The listing builds one solid part. Answer for the finished solid, in the listing's coordinates (mm). A direction names the side the tool comes from. Coordinates: 2 decimals unless noted, no trailing zeros. Order: outer loops, then holes, each group sorted by start corner. A loop starts at its lowest first (then second) coordinate and runs counter-clockwise, first axis right, second up. Notation, with made-up numbers: (-19, -5.75) -> (33, -5.75) arc R21 ccw to (33, 1.25) -> close; hole circle Ø8 at (-32.75, -18.5). An arc over 180 degrees is marked (long way). Return JSON: item names as keys, results as strings.
from build123d import *

# Parameters (mm, degrees)
F0_R     = 6
F1_DEPTH = 120
F2_R     = 3.5
F3_DEPTH = 20
F5_SIZE  = 1
F6_SIZE  = 0.5
F7_W     = 7
F7_H     = 2.68
F8_DEPTH = 12.5


with BuildPart() as f1:
    # F0 (on Front) → F1 (new body)
    with BuildSketch(Plane.XZ):
        Circle(F0_R)
    extrude(amount=F1_DEPTH)

    # F2 (on face) → F3 (cut)
    with BuildSketch(Plane.XZ.offset(120)):
        Circle(F2_R)
    extrude(amount=-F3_DEPTH, mode=Mode.SUBTRACT)

    # F5
    f5_edges = [f1.edges().sort_by_distance(p)[0] for p in [
        (-6, 0, 0),
    ]]
    chamfer(f5_edges, length=F5_SIZE)

    # F6
    f6_edges = [f1.edges().sort_by_distance(p)[0] for p in [
        (-6, -120, 0),
    ]]
    chamfer(f6_edges, length=F6_SIZE)

    # F7 (on Right) → F8 (cut, symmetric)
    with BuildSketch(Plane.YZ):
        with Locations((-96.5, 1.34)):
            Rectangle(F7_W, F7_H)
        with Locations((-96.5, -1.34)):
            Rectangle(F7_W, F7_H)
    extrude(amount=F8_DEPTH, both=True, mode=Mode.SUBTRACT)


solid = f1.part
1. For faces 4 (the face through (0, 0, 0)), 5 (the face through (0, -97, 2.68)), determine the directions among +Z, -Z, +X, -X, +Y, -Y from which every point of the face is accessible in a straight line to the end or side of a thin tool.
Answer block:
{"face 4": "+Z, -Z, +X, -X, +Y", "face 5": "+X, -X"}
2. The part is cut by section B-B on x = 0. Give the vertices of the cut face in (y, z).
Answer block:
{"outline": "(-120, -5.5) -> (-119.5, -6) -> (-1, -6) -> (0, -5) -> (0, 5) -> (-1, 6) -> (-119.5, 6) -> (-120, 5.5) -> (-120, 3.5) -> (-100, 3.5) -> (-100, 2.68) -> (-93, 2.68) -> (-93, -2.68) -> (-100, -2.68) -> (-100, -3.5) -> (-120, -3.5) -> close"}
3. Determine the mould class of faces 1 (the face through (4, -120, 0)), 2 (the face through (-6, -59, 0)), 3 (the face through (3.233, -110.14, -1.341)) for opening direction X: pulls with the +X half, pulls with the -X half, needs draft (parallel to the pull), parting line crosses it, or undercut.
Answer block:
{"face 1": "needs draft", "face 2": "parting line crosses it", "face 3": "undercut"}
4. The part is cut by section C-C on y = -97.5. Give the vertices of the cut face in (x, z).
Answer block:
{"outline": "(-5.37, -2.68) arc R6 ccw to (5.37, -2.68) -> close; (-5.37, 2.68) -> (5.37, 2.68) arc R6 ccw to start"}
5. The part is cut by section A-A on z = 0. Give the vertices of the cut face in (x, y), and give its area (3 significant figures).
Answer block:
{"outline": "(-6, -119.5) -> (-5.5, -120) -> (-3.5, -120) -> (-3.5, -100) -> (-6, -100) -> close; (-6, -93) -> (6, -93) -> (6, -1) -> (5, 0) -> (-5, 0) -> (-6, -1) -> close; (3.5, -120) -> (5.5, -120) -> (6, -119.5) -> (6, -100) -> (3.5, -100) -> close", "area": "1,210 mm2"}
6. Consider line 1 (Y direction, x = -4, z = 2.5); line 2 (Z direction, x = 0, y = -114.75). Determine where each line is inside the solid, lowest interval first. Write a range as from..to.
Answer block:
{"line 1": "y = -120..-100, -93..0", "line 2": "z = -6..-3.5, 3.5..6"}
7. Each of these flat-tipped pins is pushed along its axis until it touches: pin 1 Ø0.9 at (x, z) = (0, 3) entering from -Y; pin 2 Ø5 at (y, z) = (-54, -4) entering from -X; pin 3 Ø3 at (x, z) = (-0.5, -2) entering from +Y; pin 4 Ø3.5 at (x, y) = (2, -96.5) entering from +Z. Where does it stop, or does it pass through?
Answer block:
{"pin 1": "stops at y = -100", "pin 2": "stops at x = -5.81", "pin 3": "stops at y = 0", "pin 4": "stops at z = 5.99"}
8. The part is cut by section D-D on y = -48. Give the vertices of the cut face in (x, z).
Answer block:
{"outline": "circle Ø12 at (0, 0)"}
